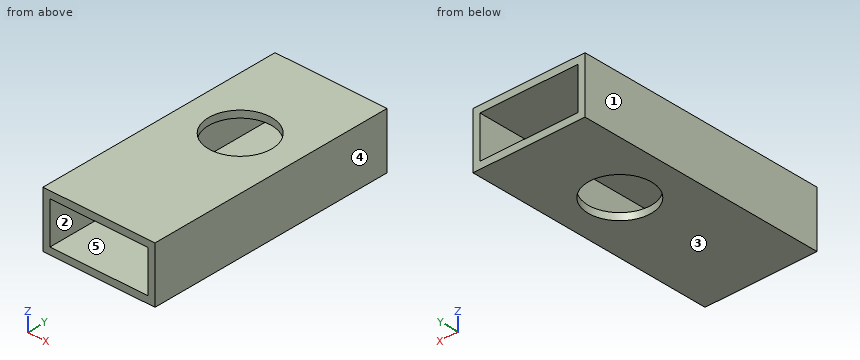
```python
from build123d import *

# Parameters (mm, degrees)
SKETCH1_W           = 50.8
SKETCH1_H           = 113.538
BOSS_EXTRUDE1_DEPTH = 25.4
SHELL1_T            = -3.175
SKETCH2_R           = 14.3129
CUT_EXTRUDE1_DEPTH  = 25.4


with BuildPart() as part:
    # Sketch1 → Boss-Extrude1 (new body)
    with BuildSketch(Plane.XY):
        Rectangle(SKETCH1_W, SKETCH1_H)
    extrude(amount=BOSS_EXTRUDE1_DEPTH)

    # Shell1
    shell1_openings = [part.faces().sort_by_distance(p)[0] for p in [
        (0, -56.769, 12.7),
        (0, 56.769, 12.7),
    ]]
    offset(amount=SHELL1_T, openings=shell1_openings, kind=Kind.INTERSECTION)

    # Sketch2 → Cut-Extrude1 (cut)
    with BuildSketch(Plane.XY.offset(25.4)):
        with Locations((0, 12.319)):
            Circle(SKETCH2_R)
    extrude(amount=-CUT_EXTRUDE1_DEPTH, mode=Mode.SUBTRACT)


solid = part.part
```
For this review, take the finished solid that the model builds, in its own axes (mm). Face numbers are marked on the shaded views. A direction names the side the tool comes from. Round coordinates to 2 decimals unless told otherwise and drop trailing zeros. Loops run counter-clockwise (first coordinate to the right, second up) from the corner with the lowest first, then second, coordinate; pieces in that order, holes last.
Q1. Insertion check: pin 1 Ø23 at (x, y) = (0, 12.319) entering from -Z; pin 2 Ø8 at (x, y) = (3.5, 2) entering from -Z. Each pin has a flat end and moves straight along its axis. Give the tip position at first contact, or say it passes through.
Result sheet:
pin 1: passes through
pin 2: stops at z = 0
Q2. Add section C-C on x = 15.5. Write out the cut boundary in (y, z) (3 decimals), plus the area to 3 significant figures.
Result sheet:
outline: (-56.769, 0) - (56.769, 0) - (56.769, 3.175) - (-56.769, 3.175) - close; (-56.769, 22.225) - (56.769, 22.225) - (56.769, 25.4) - (-56.769, 25.4) - close
area: 721 mm2
Q3. Add section B-B on z = 20.5. Write out the cut boundary in (x, y) (3 decimals).
Result sheet:
outline: (-25.4, -56.769) - (-22.225, -56.769) - (-22.225, 56.769) - (-25.4, 56.769) - close; (22.225, -56.769) - (25.4, -56.769) - (25.4, 56.769) - (22.225, 56.769) - close
Q4. Add section D-D on y = -32.5. Write out the cut boundary in (x, z) (3 decimals).
Result sheet:
outline: (-25.4, 0) - (25.4, 0) - (25.4, 25.4) - (-25.4, 25.4) - close; hole (-22.225, 3.175) - (22.225, 3.175) - (22.225, 22.225) - (-22.225, 22.225) - close
Q5. Machinability: for the marked faces 4 and 5, which of the approach directions +Z, -Z, +X, -X, +Y, -Y give a long, thin tool a straight path to every point of the face, cutting with its end or side? Answer none if there is none.
Result sheet:
face 4: +Z, -Z, +X, +Y, -Y
face 5: +Y, -Y
Q6. Mouldability with a two-part tool opening along X and no side actions: class the marked faces 1, 2 and 3 as +X half, -X half, draft (parallel to the pull), parting line (faces both ways), or undercut.
Result sheet:
face 1: -X half
face 2: undercut
face 3: draft
Q7. To check wall thickness, follow line 1 along Z through (x, y) = (16.5, -20) (3 decimals); line 2 along X through (y, z) = (38.5, 5.25) (3 decimals); line 3 along Y through (x, z) = (0, 1.1). State the ranges of each line that lie inside material, in increasing order.
Result sheet:
line 1: z = 0 to 3.175, 22.225 to 25.4
line 2: x = -25.4 to -22.225, 22.225 to 25.4
line 3: y = -56.77 to -1.99, 26.63 to 56.77
Q8. Add section A-A on x = 0. Write out the cut boundary in (y, z) (3 decimals).
Result sheet:
outline: (-56.769, 0) - (-1.994, 0) - (-1.994, 3.175) - (-56.769, 3.175) - close; (-56.769, 22.225) - (-1.994, 22.225) - (-1.994, 25.4) - (-56.769, 25.4) - close; (26.632, 0) - (56.769, 0) - (56.769, 3.175) - (26.632, 3.175) - close; (26.632, 22.225) - (56.769, 22.225) - (56.769, 25.4) - (26.632, 25.4) - close
